Geometry: final body of the model. Coordinates: model frame, mm. Face numbers are marked on the shaded views. A direction names the side the tool comes from. Round coordinates to 2 decimals unless told otherwise and drop trailing zeros. Order: outer loops, then holes, each group sorted by start corner. A loop starts at its lowest first (then second) coordinate and runs counter-clockwise, first axis right, second up. Notation, with made-up numbers: (67, -19.75) -> (114, -19.75) arc R18 ccw to (114, 12.25) -> close; hole circle Ø9 at (45, 54.5). An arc over 180 degrees is marked (long way). Put each result on its own line as item: value.
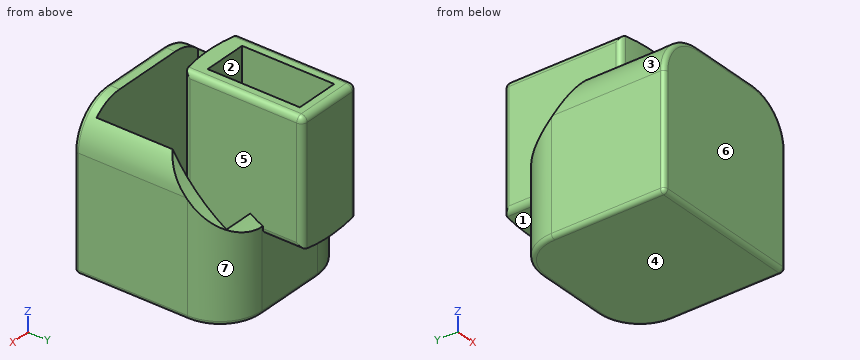
```python
from build123d import *

# Parameters (mm, degrees)
F0_W         = 18.5
F0_H         = 18.5
F1_DEPTH     = 18.5
F2_R         = 19
F3_DEPTH     = 25.4
F4_T         = -1.5
F6_DEPTH     = 14
F7_T         = 1.5
F7_T3_DEPTH  = 3.8130317325
F7_T5_DEPTH  = 20
F7_T7_DEPTH  = 18.5
F7_T9_DEPTH  = 12.1348502244
F7_T11_DEPTH = 18.5
F7_T13_DEPTH = 4.6348502244
F7_T16_ANGLE = 5.1594967302
F7_T18_ANGLE = 27.6449084771
F7_T20_ANGLE = 5.1594967302
F7_T22_ANGLE = 27.6449084771
F9_DEPTH     = 23.32034
F10_DEPTH    = 8.55107
F11_R        = 5
F12_R        = 0.7
F13_R        = 0.5


# Not quite as in the source:
# - a shell that OpenCascade refuses in one call is made with other operations: the cavity is built on its own and cut out


with BuildPart() as f1:
    # F0 (on Top) → F1 (new body)
    with BuildSketch(Plane.XY):
        Rectangle(F0_W, F0_H)
    extrude(amount=-F1_DEPTH)

    # F2 (on face) → F3 (cut)
    with BuildSketch(Plane.YZ.offset(9.25)):
        with Locations((17.6200576851, 8.3700576851)):
            Circle(F2_R)
    extrude(amount=-F3_DEPTH, mode=Mode.SUBTRACT)

    # F4
    f4_openings = [f1.faces().sort_by_distance(p)[0] for p in [
        (0, -4.343484, 0),
        (0, 4.185029, -5.064971),
    ]]
    offset(amount=F4_T, openings=f4_openings)

    # F5 (on Front) → F6 (join)
    with BuildSketch(Plane.XZ):
        with BuildLine():
            Line((4.125, -9.5), (4.125, 5))
            Line((4.125, 5), (0, 5))
            Line((0, 5), (-4.125, 5))
            Line((-4.125, 5), (-4.125, -9.5))
            ThreePointArc((-4.125, -9.5), (0, -10), (4.125, -9.5))
        make_face()
    extrude(amount=-F6_DEPTH)

    # F7: shell of thickness 1.5, made by hand


with BuildPart() as f7_core1:
    # F7_t2: copy of F1
    add(f1.part)

    # the walls: a layer under each face that stays
    f7_faces = [f7_core1.faces().sort_by_distance(p)[0] for p in [
        (9.25, 0, -9.25),
        (-7.9285714286, -8.549069162, 0),
        (8.3958333333, 1.5822898542, -1.8176801895),
        (0, 9.25, -13.5934841338),
        (0, 0, -18.5),
        (0, -9.25, -9.25),
        (-8.3958333333, 1.5822898542, -1.8176801895),
        (-9.25, 0, -9.25),
        (7.75, 0, -8.5),
        (0, -7.75, -8.5),
        (-7.75, 0, -8.5),
        (4.125, 7, -2.25),
        (0, 7.75, -12.4325748878),
        (0, 11.625, -10),
        (-4.125, 7, -2.25),
        (0, 0, -17),
        (0, 0, -2.5),
        (0, 14, -2.5),
        (0, 3.875, -10),
    ]]
    thicken(f7_faces, amount=-F7_T, mode=Mode.SUBTRACT)

    # F7_s4 → F7_t3 (cut)
    with BuildSketch(Plane.XY.offset(-11)):
        Polygon((4.14, 9.265), (4.125, 7.75), (2.625, 7.75), (2.625, 9.25), align=None)
        Polygon((-4.14, 9.265), (-4.125, 7.75), (-2.625, 7.75), (-2.625, 9.25), align=None)
    extrude(amount=F7_T3_DEPTH, mode=Mode.SUBTRACT)

    # F7_s6 → F7_t5 (cut)
    with BuildSketch(Plane.XY.offset(-18.5)):
        Polygon((7.735, -7.735), (9.25, -7.75), (9.25, -9.25), (7.75, -9.25), align=None)
        Polygon((-7.735, -7.735), (-7.75, -9.25), (-9.25, -9.25), (-9.25, -7.75), align=None)
    extrude(amount=F7_T5_DEPTH, mode=Mode.SUBTRACT)

    # F7_s8 → F7_t7 (cut)
    with BuildSketch(Plane.XZ.offset(-9.25)):
        Polygon((7.735, -16.985), (9.25, -17), (9.25, -18.5), (7.75, -18.5), align=None)
        Polygon((-7.735, -16.985), (-9.25, -17), (-9.25, -18.5), (-7.75, -18.5), align=None)
    extrude(amount=F7_T7_DEPTH, mode=Mode.SUBTRACT)

    # F7_s10 → F7_t9 (cut)
    with BuildSketch(Plane.XY.offset(-18.5)):
        Polygon((7.735, 7.735), (9.25, 7.75), (9.25, 9.25), (7.75, 9.25), align=None)
        Polygon((-7.735, 7.735), (-9.25, 7.75), (-9.25, 9.25), (-7.75, 9.25), align=None)
    extrude(amount=F7_T9_DEPTH, mode=Mode.SUBTRACT)

    # F7_s12 → F7_t11 (cut)
    with BuildSketch(Plane.YZ.offset(-9.25)):
        Polygon((-7.735, -16.985), (-9.25, -17), (-9.25, -18.5), (-7.75, -18.5), align=None)
        Polygon((7.735, -16.985), (9.25, -17), (9.25, -18.5), (7.75, -18.5), align=None)
    extrude(amount=F7_T11_DEPTH, mode=Mode.SUBTRACT)

    # F7_s14 → F7_t13 (cut)
    with BuildSketch(Plane.XY.offset(-11)):
        Polygon((4.14, 7.735), (2.625, 7.75), (2.625, 9.25), (4.125, 9.25), align=None)
        Polygon((-4.14, 7.735), (-4.125, 9.25), (-2.625, 9.25), (-2.625, 7.75), align=None)
    extrude(amount=F7_T13_DEPTH, mode=Mode.SUBTRACT)

    # F7_s15 → F7_t16 (revolve, cut)
    with BuildSketch(Plane(origin=(0, 9.1498364132, -5.5625660113), x_dir=(1, 0, 0), z_dir=(0, -0.8544846032, 0.5194767203))):
        Polygon((4.14, -2.679704803), (4.125, -4.194704803), (2.625, -4.194704803), (2.625, -2.694704803), align=None)
    revolve(axis=Axis((4.125, 17.6200576851, 8.3700576851), (1, 0, 0)), revolution_arc=F7_T16_ANGLE, mode=Mode.SUBTRACT)

    # F7_s17 → F7_t18 (revolve, cut)
    with BuildSketch(Plane(origin=(-1.6855904875, 0, 0.4147212383), x_dir=(0, 1, 0), z_dir=(-0.971040724, 0, 0.2389140271))):
        Polygon((9.265, 10.2254072398), (7.75, 10.2104072398), (7.75, 8.7104072398), (9.25, 8.7104072398), align=None)
    revolve(axis=Axis((0, 9.25, 7.265625), (0, -1, 0)), revolution_arc=F7_T18_ANGLE, mode=Mode.SUBTRACT)

    # F7_s19 → F7_t20 (revolve, cut)
    with BuildSketch(Plane(origin=(0, 9.1498364132, -5.5625660113), x_dir=(1, 0, 0), z_dir=(0, -0.8544846032, 0.5194767203))):
        Polygon((-4.14, -2.679704803), (-4.125, -4.194704803), (-2.625, -4.194704803), (-2.625, -2.694704803), align=None)
    revolve(axis=Axis((-4.125, 17.6200576851, 8.3700576851), (1, 0, 0)), revolution_arc=F7_T20_ANGLE, mode=Mode.SUBTRACT)

    # F7_s21 → F7_t22 (revolve, cut)
    with BuildSketch(Plane(origin=(-1.6855904875, 0, 0.4147212383), x_dir=(0, 1, 0), z_dir=(-0.971040724, 0, 0.2389140271))):
        Polygon((7.735, 10.2254072398), (9.25, 10.2104072398), (9.25, 8.7104072398), (7.75, 8.7104072398), align=None)
    revolve(axis=Axis((0, 7.75, 7.265625), (0, -1, 0)), revolution_arc=F7_T22_ANGLE, mode=Mode.SUBTRACT)


with BuildPart() as f1_1:
    add(f1.part)

    # what is left inside the walls is the cavity
    f7_cavity = [f7_core1.part.solids().sort_by_distance(p)[0] for p in [
        (-2.61, 7, 0.573356),
    ]]
    add(f7_cavity, mode=Mode.SUBTRACT)

    # F8 (on face) → F9 (join)
    with BuildSketch(Plane.XY.offset(5)):
        with BuildLine():
            Line((4.125, 0), (-4.125, 0))
            ThreePointArc((-4.125, 0), (0, -0.5), (4.125, 0))
        make_face()
    extrude(amount=-F9_DEPTH)

    # F10 (add): a face of the model
    f10_faces = [f1_1.faces().sort_by_distance(p)[0] for p in [
        (0, 0, -13.4156113664),
    ]]
    extrude(f10_faces, amount=F10_DEPTH)

    # F11
    f11_edges = [f1_1.edges().sort_by_distance(p)[0] for p in [
        (-9.25, -4.343484, 0),
        (9.25, -4.343484, 0),
        (9.25, 9.25, -13.593484),
        (-9.25, 9.25, -13.593484),
    ]]
    fillet(f11_edges, radius=F11_R)

    # F12
    f12_edges = [f1_1.edges().sort_by_distance(p)[0] for p in [
        (4.125, 14, -2.25),
        (-4.125, 14, -2.25),
        (4.125, 7, 5),
        (-4.125, 7, 5),
        (-4.125, 11.625, -9.5),
        (4.125, 11.625, -9.5),
        (4.125, 0, -6),
        (-4.125, 0, -6),
        (0, 14, 5),
    ]]
    fillet(f12_edges, radius=F12_R)

    # F13
    f13_edges = [f1_1.edges().sort_by_distance(p)[0] for p in [
        (9.25, -2.5, -18.5),
        (0, -9.25, -18.5),
        (9.25, -9.25, -11.75),
        (-9.25, -2.5, -18.5),
        (-9.25, -9.25, -11.75),
        (0, 9.25, -18.5),
        (7.785534, 7.785534, -18.5),
        (-7.785534, 7.785534, -18.5),
        (7.785534, -9.25, -1.464466),
        (-7.785534, -9.25, -1.464466),
        (0, -9.25, 0),
    ]]
    fillet(f13_edges, radius=F13_R)


solid = f1_1.part
```
1. Set-up query: the marked faces 1, 2 and 3. Return all of +Z, -Z, +X, -X, +Y, -Y with unobstructed straight access to the full face (end or side cutting, diameter ignored); none if empty.
Ans:
face 1: -Z, +Y
face 2: +Z
face 3: +Z, -X, +Y, -Y
2. Cut plane C-C on z = 1. Return loops of the section in (x, y) (3 decimals).
Ans:
outline: (-4.125, 0.558) arc R0.7 ccw to (-3.57, -0.127) arc R17.266 ccw to (3.57, -0.127) arc R0.7 ccw to (4.125, 0.558) -> (4.125, 13.3) arc R0.7 ccw to (3.425, 14) -> (-3.425, 14) arc R0.7 ccw to (-4.125, 13.3) -> close; hole (-2.625, 1.5) -> (2.625, 1.5) -> (2.625, 12.5) -> (-2.625, 12.5) -> close
3. Contact query for flat-ended pins moving along their axis: P1, Ø3, axis at x = -1, y = 10.5, coming from the -Z side; P2, Ø1.5, axis at y = 9.5, z = -5.5, coming from the -X side (3 decimals); P3, Ø0.5, axis at x = -1, y = -8, coming from the +Z side. Output: stop coordinate, or through.
Ans:
P1: z = -18.43
P2: x = -4.125
P3: z = 0
4. Cut plane D-D on x = -0.25. Return loops of the section in (y, z).
Ans:
outline: (-9.25, -18) arc R0.5 ccw to (-8.75, -18.5) -> (8.75, -18.5) arc R0.5 ccw to (9.25, -18) -> (9.25, -10) -> (14, -10) -> (14, 4.3) arc R0.7 ccw to (13.3, 5) -> (12.5, 5) -> (12.5, -8.5) -> (1.5, -8.5) -> (1.5, 5) -> (-0.5, 5) -> (-0.5, -17) -> (-7.75, -17) -> (-7.75, 0) -> (-8.75, 0) arc R0.5 ccw to (-9.25, -0.5) -> close
5. Cut plane A-A on z = -7.5. Return loops of the section in (x, y) (3 decimals).
Ans:
outline: (-9.25, -8.75) arc R0.5 ccw to (-8.75, -9.25) -> (8.75, -9.25) arc R0.5 ccw to (9.25, -8.75) -> (9.25, 4.25) arc R5 ccw to (8.307, 7.173) -> (7.75, 7.173) -> (7.75, -7.75) -> (-7.75, -7.75) -> (-7.75, 7.173) -> (-8.307, 7.173) arc R5 ccw to (-9.25, 4.25) -> close; (-4.125, 0.558) arc R0.7 ccw to (-3.57, -0.127) arc R17.266 ccw to (3.57, -0.127) arc R0.7 ccw to (4.125, 0.558) -> (4.125, 13.3) arc R0.7 ccw to (3.425, 14) -> (-3.425, 14) arc R0.7 ccw to (-4.125, 13.3) -> close; hole (-2.625, 1.5) -> (2.625, 1.5) -> (2.625, 12.5) -> (-2.625, 12.5) -> close
6. Draft query along Y for the marked faces 4, 5, 6 and 7. Return one class per face: +Y half, -Y half, draft (parallel to the pull), parting line (faces both ways), or undercut.
Ans:
face 4: draft
face 5: undercut
face 6: -Y half
face 7: +Y half
7. Cut plane B-B on y = -2. Return loops of the section in (x, z), and give its area (3 significant figures).
Ans:
outline: (-9.25, -18) arc R0.5 ccw to (-8.75, -18.5) -> (8.75, -18.5) arc R0.5 ccw to (9.25, -18) -> (9.25, -5) arc R5 ccw to (7.75, -1.43) -> (7.75, -17) -> (-7.75, -17) -> (-7.75, -1.43) arc R5 ccw to (-9.25, -5) -> close
area: 71.0 mm²
8. Material intervals for probe 1 along X at (y, z) = (4, -5.5) (3 decimals); probe 2 along X at (y, z) = (4.5, -16.25) (3 decimals); probe 3 along Y at (x, z) = (0, -6.75), sorted ascending.
Ans:
probe 1: -9.25 to -7.75, -4.125 to -2.625, 2.625 to 4.125, 7.75 to 9.25
probe 2: -9.244 to -7.75, -4.125 to 4.125, 7.75 to 9.244
probe 3: -9.25 to -7.75, -0.5 to 1.5, 12.5 to 14
